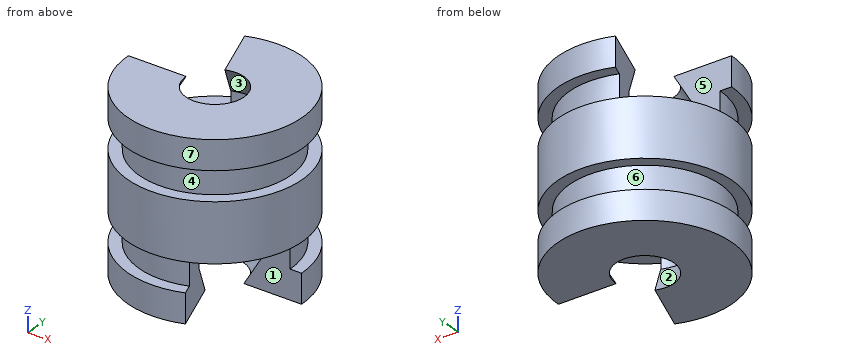
from build123d import *

# Parameters (mm, degrees)
SKETCH001_W  = 16
SKETCH001_H  = 16
GROOVE_ANGLE = -70


with BuildPart() as part:
    # Sketch (on XZ_Plane of Origin) → Revolution (revolve)
    with BuildSketch(Plane.XZ):
        Polygon((-5, 15), (-15, 15), (-15, 10), (-13, 10), (-13, 5), (-15, 5), (-15, -5), (-13, -5), (-13, -10), (-15, -10), (-15, -15), (-5, -15), (-8, -10), (-8, 10), align=None)
    revolve(axis=Axis((0, 0, 0), (0, 0, 1)))

    # Sketch001 (on XZ_Plane of Origin) → Groove (revolve, cut)
    with BuildSketch(Plane.XZ):
        with Locations((-8, 13)):
            Rectangle(SKETCH001_W, SKETCH001_H)
        with Locations((8, -13)):
            Rectangle(SKETCH001_W, SKETCH001_H)
    revolve(axis=Axis((0, 0, 0), (0, 0, 1)), revolution_arc=GROOVE_ANGLE, mode=Mode.SUBTRACT)


solid = part.part
Here's how the part is built. I have some questions about the finished solid (model axes, mm). Face numbers are marked on the shaded views. A direction names the side the tool comes from. Round coordinates to 2 decimals unless told otherwise and drop trailing zeros. Order: outer loops, then holes, each group sorted by start corner. A loop starts at its lowest first (then second) coordinate and runs counter-clockwise, first axis right, second up. Notation, with made-up numbers: M 58.5,89.5 L 63.5,89.5 A11 ccw 63.5,100.5 Z; hole C -17,-13 d9. An arc over 180 degrees is marked long. Return JSON: item names as keys, results as strings. Group by question number.
1. Please list where these lines run through material, in increasing order: probe 1 along X at (y, z) = (0, -0.75); probe 2 along Z at (x, y) = (-4.75, -12.5).
2. If we mould it in two halves opening along Y, with no side actions, what happens to the marked faces 1, 2, 3 and 4? For each: pulls with the +Y half, pulls with the -Y half, needs draft (parallel to the pull), parting line crosses it, or undercut.
3. I'm going to push flat-ended pins straight in: pin 1 Ø1.5 at (y, z) = (8.5, -4.5) entering from -X; pin 2 Ø8 at (x, z) = (7.5, 5.5) entering from +Y; pin 3 Ø3 at (x, z) = (-11, 8.5) entering from +Y. Where does each tip first touch, or does it pass through?
4. If we section it at D-D on z = 12: List the corners of the cut face in (x, y) for me.
5. If we section it at B-B on z = 4.5: List the corners of the cut face in (x, y) for me, then the cut area to 3 significant figures.
6. If we section it at C-C on x = -10.25: List the corners of the cut face in (y, z) for me.
7. If we section it at A-A on x = 0: List the corners of the cut face in (y, z) for me.
8. On a 3-axis mill with a long thin cutter (end or side, diameter ignored), from which of +Z, -Z, +X, -X, +Y, -Y can I reach the whole of each face in a straight line? I mean the marked faces 5, 6 and 7. Say none if no direction works.
Reply:
{
 "1": {"probe 1": "-15 to -8, 8 to 15", "probe 2": "-15 to -10, -5 to 5, 10 to 15"},
 "2": {"face 1": "pulls with the -Y half", "face 2": "undercut", "face 3": "undercut", "face 4": "parting line crosses it"},
 "3": {"pin 1": "x = -12.84", "pin 2": "y = 14.58", "pin 3": "y = 0"},
 "4": {"outline": "M -15,0 A15 ccw long -5.13,14.1 L -2.33,6.39 A6.8 cw long -6.8,0 Z"},
 "5": {"outline": "C 0,0 d30; hole C 0,0 d16", "area": "506 mm^2"},
 "6": {"outline": "M -10.95,-15 L 10.95,-15 L 10.95,-10 L 8,-10 L 8,-5 L 10.95,-5 L 10.95,5 L 0,5 L 0,15 L -10.95,15 L -10.95,10 L -8,10 L -8,5 L -10.95,5 L -10.95,-5 L -8,-5 L -8,-10 L -10.95,-10 Z"},
 "7": {"outline": "M -15,-15 L -5,-15 L -8,-10 L -8,10 L -5,15 L -15,15 L -15,10 L -13,10 L -13,5 L -15,5 L -15,-5 L -13,-5 L -13,-10 L -15,-10 Z; M 5,-15 L 15,-15 L 15,-10 L 13,-10 L 13,-5 L 15,-5 L 15,5 L 13,5 L 13,10 L 15,10 L 15,15 L 5,15 L 8,10 L 8,-10 Z"},
 "8": {"face 5": "+Z, -X, +Y", "face 6": "none", "face 7": "+Z, -Z"}
}
